Can you work these out from the model? Positions are in its coordinate system, mm. A direction names the side the tool comes from. Coordinates: 2 decimals unless noted, no trailing zeros. Order: outer loops, then holes, each group sorted by start corner. A loop starts at its lowest first (then second) coordinate and runs counter-clockwise, first axis right, second up. Notation, with made-up numbers: M 12.25,3 L 44.25,3 A11 ccw 44.25,21 Z; hole C 34,0 d3. An arc over 180 degrees is marked long. Answer as CSV lines item,"result". Start each with the question number.
1. If we section it at B-B (y = 31): List the corners of the cut face in (x, z) for me.
2. If we section it at C-C (x = 29.5): List the corners of the cut face in (y, z) for me.
3. If we section it at A-A (y = 49.5): List the corners of the cut face in (x, z) for me.
4. I need wall thicknesses on line 1 along Y through (x, z) = (0, 0.8); line 2 along X through (y, z) = (32.5, 7.5); line 3 along Y through (x, z) = (-10.5, 8.75). Which ranges of each line are inside material? Lowest first, please. Write a range as from..to.
5. If we mould it in two halves opening along X, with no side actions, what happens to faces 4 (the face through (35.01, -74.56, 5.39)), 5 (the face through (0, 76, 5)), 6 (the face through (-35.063, 75.562, 5.374))? For each: released by +X, released by -X, zero draft, split by the parting line, or undercut.
6. On a 3-axis mill with a long thin cutter (end or side, diameter ignored), from which of +Z, -Z, +X, -X, +Y, -Y can I reach the whole of each face in a straight line? I mean faces 1 (the face through (-39, 1, 5)), 2 (the face through (-9.145, 75.507, 5.604)), 3 (the face through (0, -75, 5)). Say none if no direction works.
7. Will these pins go through, and if not, where does the flat tip stop? pin 1 (0.8 mm diameter, centred on x = 38.5, z = 5.5, fed in from -Y); pin 2 (1 mm diameter, centred on x = -10, y = 42, fed in from +Z); pin 3 (8 mm diameter, centred on x = -2, y = 13, fed in from -Z); pin 4 (0.7 mm diameter, centred on x = 8.5, z = 10.5, fed in from -Y).
8. If we section it at D-D (x = 0): Give the number of separate pieces and of enclosed holes in the cut face, plus the area to 3 significant figures.
```python
from build123d import *

# Parameters (mm, degrees)
F0_W        = 12
F0_H        = 4
F0_R        = 2.5
F0_R_2      = 7
F1_DEPTH    = 1
F3_DEPTH    = 8.9
F5_DEPTH    = 1
F6_T1_DEPTH = 155
F6_T3_DEPTH = 79
F6_T5_DEPTH = 11.2553390593
F6_T7_DEPTH = 15.2364770085
F7_SIZE     = 0.4
F8_W        = 13.5
F8_H        = 4
F8_W_2      = 24
F9_DEPTH    = 25
F10_R       = 3.5
F10_W       = 17
F10_H       = 5.5
F11_DEPTH   = 25
F12_R       = 2
F13_DEPTH   = 25


# Not quite as in the source:
# - a fillet or chamfer that OpenCascade refuses, or shapes differently, is made with other operations: its cross-section is extruded or revolved along the edge and cut away or added
# - a feature names something its author has since deleted; it is built from what else it names


with BuildPart() as f1:
    # F0 (on Top) → F1 (new body)
    with BuildSketch(Plane.XY):
        Polygon((32, 76), (-32, 76), (-39, 75), (-39, -75), (-32, -76), (32, -76), (39, -75), (39, 75), align=None)
        with Locations((0, -63)):
            Rectangle(F0_W, F0_H, mode=Mode.SUBTRACT)
        with Locations((0, 49.5)):
            Circle(F0_R, mode=Mode.SUBTRACT)
        with Locations((0, 60)):
            Circle(F0_R_2, mode=Mode.SUBTRACT)
    extrude(amount=F1_DEPTH)

    # F2 (on face) → F3 (join)
    with BuildSketch(Plane.XY.offset(1)):
        Polygon((39, 75), (32, 76), (-32, 76), (-39, 75), (-39, -75), (-32, -76), (32, -76), (39, -75), align=None)
        Polygon((31.9289321881, -75), (-31.9289321881, -75), (-38, -74.1327045983), (-38, 74.1327045983), (-31.9289321881, 75), (31.9289321881, 75), (38, 74.1327045983), (38, -74.1327045983), align=None, mode=Mode.SUBTRACT)
    extrude(amount=F3_DEPTH)

    # F4 (on face) → F5 (join)
    with BuildSketch(Plane.XY.offset(9.9)):
        Polygon((39, -75), (39, 75), (32, 76), (-32, 76), (-39, 75), (-39, -75), (-32, -76), (32, -76), align=None)
        Polygon((38, -74.1327045983), (31.9289321881, -75), (-31.9289321881, -75), (-38, -74.1327045983), (-38, 74.1327045983), (-31.9289321881, 75), (31.9289321881, 75), (38, 74.1327045983), align=None, mode=Mode.SUBTRACT)
        Polygon((-31.9289321881, -75), (31.9289321881, -75), (38, -74.1327045983), (38, 74.1327045983), (31.9289321881, 75), (-31.9289321881, 75), (-38, 74.1327045983), (-38, -74.1327045983), align=None)
        Polygon((-37, 73.2654091966), (-31.8578643763, 74), (31.8578643763, 74), (37, 73.2654091966), (37, -73.2654091966), (31.8578643763, -74), (-31.8578643763, -74), (-37, -73.2654091966), align=None, mode=Mode.SUBTRACT)
    extrude(amount=F5_DEPTH)

    # F6: fillet of radius 1 on 16 edges, made by hand

    # F6_s2 → F6_t1 (cut)
    with BuildSketch(Plane.XZ.offset(-77.5)):
        with BuildLine():
            ThreePointArc((-39, 9.9), (-38.7071067812, 10.6071067812), (-38, 10.9))
            Line((-38, 10.9), (-39, 10.9))
            Line((-39, 10.9), (-39, 9.9))
        make_face()
        with BuildLine():
            ThreePointArc((39, 9.9), (38.7071067812, 10.6071067812), (38, 10.9))
            Line((38, 10.9), (39, 10.9))
            Line((39, 10.9), (39, 9.9))
        make_face()
        with BuildLine():
            ThreePointArc((38, 0), (38.7071067812, 0.2928932188), (39, 1))
            Line((39, 1), (39, 0))
            Line((39, 0), (38, 0))
        make_face()
        with BuildLine():
            ThreePointArc((-38, 0), (-38.7071067812, 0.2928932188), (-39, 1))
            Line((-39, 1), (-39, 0))
            Line((-39, 0), (-38, 0))
        make_face()
    extrude(amount=F6_T1_DEPTH, mode=Mode.SUBTRACT)

    # F6_s4 → F6_t3 (cut)
    with BuildSketch(Plane.YZ.offset(-39.5)):
        with BuildLine():
            ThreePointArc((76, 9.9), (75.7071067812, 10.6071067812), (75, 10.9))
            Line((75, 10.9), (76, 10.9))
            Line((76, 10.9), (76, 9.9))
        make_face()
        with BuildLine():
            ThreePointArc((-76, 9.9), (-75.7071067812, 10.6071067812), (-75, 10.9))
            Line((-75, 10.9), (-76, 10.9))
            Line((-76, 10.9), (-76, 9.9))
        make_face()
        with BuildLine():
            ThreePointArc((-75, 0), (-75.7071067812, 0.2928932188), (-76, 1))
            Line((-76, 1), (-76, 0))
            Line((-76, 0), (-75, 0))
        make_face()
        with BuildLine():
            ThreePointArc((76, 1), (75.7071067812, 0.2928932188), (75, 0))
            Line((75, 0), (76, 0))
            Line((76, 0), (76, 1))
        make_face()
    extrude(amount=F6_T3_DEPTH, mode=Mode.SUBTRACT)

    # F6_s6 → F6_t5 (cut)
    with BuildSketch(Plane.XY.offset(-0.1776695297)):
        with BuildLine():
            ThreePointArc((31.9289321881, 76), (31.9998212082, 75.9974842088), (32.0703535444, 75.9899494937))
            Line((32.0703535444, 75.9899494937), (32, 76))
            Line((32, 76), (31.9289321881, 76))
        make_face()
        with BuildLine():
            ThreePointArc((-31.9289321881, 76), (-31.9998212082, 75.9974842088), (-32.0703535444, 75.9899494937))
            Line((-32.0703535444, 75.9899494937), (-32, 76))
            Line((-32, 76), (-31.9289321881, 76))
        make_face()
        with BuildLine():
            ThreePointArc((32.0703535444, -75.9899494937), (31.9998212082, -75.9974842088), (31.9289321881, -76))
            Line((31.9289321881, -76), (32, -76))
            Line((32, -76), (32.0703535444, -75.9899494937))
        make_face()
        with BuildLine():
            ThreePointArc((-31.9289321881, -76), (-31.9998212082, -75.9974842088), (-32.0703535444, -75.9899494937))
            Line((-32.0703535444, -75.9899494937), (-32, -76))
            Line((-32, -76), (-31.9289321881, -76))
        make_face()
    extrude(amount=F6_T5_DEPTH, mode=Mode.SUBTRACT)

    # F6_s8 → F6_t7 (cut)
    with BuildSketch(Plane.XY.offset(-2.1682385042)):
        with BuildLine():
            ThreePointArc((39, -74.1327045983), (38.755453955, -74.7879063397), (38.1414213562, -75.122654092))
            Line((38.1414213562, -75.122654092), (39, -75))
            Line((39, -75), (39, -74.1327045983))
        make_face()
        with BuildLine():
            ThreePointArc((39, 74.1327045983), (38.755453955, 74.7879063397), (38.1414213562, 75.122654092))
            Line((38.1414213562, 75.122654092), (39, 75))
            Line((39, 75), (39, 74.1327045983))
        make_face()
        with BuildLine():
            ThreePointArc((-38.1414213562, -75.122654092), (-38.755453955, -74.7879063397), (-39, -74.1327045983))
            Line((-39, -74.1327045983), (-39, -75))
            Line((-39, -75), (-38.1414213562, -75.122654092))
        make_face()
        with BuildLine():
            ThreePointArc((-39, 74.1327045983), (-38.755453955, 74.7879063397), (-38.1414213562, 75.122654092))
            Line((-38.1414213562, 75.122654092), (-39, 75))
            Line((-39, 75), (-39, 74.1327045983))
        make_face()
    extrude(amount=F6_T7_DEPTH, mode=Mode.SUBTRACT)

    # F7
    f7_edges = [f1.edges().sort_by_distance(p)[0] for p in [
        (-34.428932, 73.632705, 9.9),
        (-37, 0, 9.9),
        (0, 74, 9.9),
        (34.428932, 73.632705, 9.9),
        (37, 0, 9.9),
        (34.428932, -73.632705, 9.9),
        (0, -74, 9.9),
        (-34.428932, -73.632705, 9.9),
    ]]
    chamfer(f7_edges, length=F7_SIZE)

    # F8 (on face) → F9 (cut)
    with BuildSketch(Plane.YZ.offset(39)):
        with Locations((14.3827045983, 5.45)):
            Rectangle(F8_W, F8_H)
        with Locations((39.1327045983, 5.45)):
            Rectangle(F8_W_2, F8_H)
    extrude(amount=-F9_DEPTH, mode=Mode.SUBTRACT)

    # F10 (on face) → F11 (cut)
    with BuildSketch(Plane(origin=(0, 76, 0), x_dir=(-1, 0, 0), z_dir=(0, 1, 0))):
        with Locations((12.6414213562, 5.45)):
            Circle(F10_R)
        with Locations((-13.6414213562, 5.25)):
            Rectangle(F10_W, F10_H)
    extrude(amount=-F11_DEPTH, mode=Mode.SUBTRACT)

    # F12 (on face) → F13 (cut)
    with BuildSketch(Plane.XZ.offset(76)):
        with Locations((8.1414213562, 5.45)):
            Circle(F12_R)
    extrude(amount=-F13_DEPTH, mode=Mode.SUBTRACT)


solid = f1.part
```
Solved:
1,outline,"M -39,1 A1 ccw -38,0 L 38,0 A1 ccw 39,1 L 39,3.45 L 38,3.45 L 38,1 L -38,1 L -38,9.9 L -37.4,9.9 L -37,10.3 L -37,10.9 L -38,10.9 A1 ccw -39,9.9 Z; M 37,10.3 L 37.4,9.9 L 38,9.9 L 38,7.45 L 39,7.45 L 39,9.9 A1 ccw 38,10.9 L 37,10.9 Z"
2,outline,"M -76,1 A1 ccw -75,0 L 75,0 A1 ccw 76,1 L 76,9.9 A1 ccw 75,10.9 L 74,10.9 L 74,10.3 L 74.4,9.9 L 75,9.9 L 75,1 L -75,1 L -75,9.9 L -74.4,9.9 L -74,10.3 L -74,10.9 L -75,10.9 A1 ccw -76,9.9 Z"
3,outline,"M -39,1 A1 ccw -38,0 L -2.5,0 L -2.5,1 L -38,1 L -38,9.9 L -37.4,9.9 L -37,10.3 L -37,10.9 L -38,10.9 A1 ccw -39,9.9 Z; M 2.5,0 L 38,0 A1 ccw 39,1 L 39,3.45 L 38,3.45 L 38,1 L 2.5,1 Z; M 37,10.3 L 37.4,9.9 L 38,9.9 L 38,7.45 L 39,7.45 L 39,9.9 A1 ccw 38,10.9 L 37,10.9 Z"
4,line 1,"-75.98..-65, -61..47, 52..53, 67..75.98"
4,line 2,"-39..-38, 38..39"
4,line 3,"-76..-75, 75..76"
5,face 4,"undercut"
5,face 5,"zero draft"
5,face 6,"released by -X"
6,face 1,"+Z, -Z, -X, +Y, -Y"
6,face 2,"+Y"
6,face 3,"none"
7,pin 1,"y = -75.13"
7,pin 2,"z = 1"
7,pin 3,"z = 0"
7,pin 4,"y = -75.97"
8,separate pieces,"4"
8,enclosed holes,"0"
8,area,"150 mm²"
